Input: part model. Units: mm. Frame: model coordinates. Give positions to 0.01 mm unless a question says otherwise; leave off trailing zeros. Answer in a Markdown table with one row per item. Add a question column.
1. Ray query, line 1 (Y direction, x = -75, z = 11.5); line 2 (Z direction, x = -66, y = -19); line 3 (X direction, y = 1, z = 3.5). Return the intervals inside material, ascending. Write a range as [from, to].
2. Mould query, pull axis X, two halves, no side actions, for faces 1 (the face through (110, 5, 2)), 2 (the face through (-3, -40, 0)). Classes: released by +X, released by -X, zero draft, split by the parting line, or undercut.
3. Contact query for flat-ended pins moving along their axis: pin 1 (1.5 mm diameter, centred on x = -92, y = -22.5, fed in from +Z); pin 2 (8 mm diameter, centred on x = 65, z = -77.5, fed in from +Y); pin 3 (10 mm diameter, centred on x = -88, y = -4, fed in from +Z). Output: stop coordinate, or through.
```python
from build123d import *


with BuildPart() as part:
    # 草图2 → 放样1 section 0
    with BuildSketch(Plane(origin=(0, 0, 0), x_dir=(1, 0, 0), z_dir=(0, 1, 0))):
        with BuildLine():
            Line((-115, -115), (-115, 115))
            Line((-115, 115), (115, 115))
            Line((115, 115), (115, -115))
            Line((115, -115), (-115, -115))
        make_face()
    # 草图3 → 放样1 section 1
    with BuildSketch(Plane(origin=(0, -40, 0), x_dir=(1, 0, 0), z_dir=(0, 1, 0))):
        with BuildLine():
            Line((125, -125), (125, 125))
            Line((125, 125), (-125, 125))
            Line((-125, 125), (-125, -125))
            Line((-125, -125), (125, -125))
        make_face()
    loft()

    # 扫描1: sweep along a path in 草图2<2>
    with BuildLine(Plane(origin=(0, 0, 0), x_dir=(1, 0, 0), z_dir=(0, 1, 0))) as sweep_1_path:
        Line((-115, -115), (-115, 115))
        Line((-115, 115), (115, 115))
        Line((115, 115), (115, -115))
        Line((115, -115), (-115, -115))
    # 草图4 → 扫描1 (sweep)
    with BuildSketch(Plane(origin=(0, 0, 115), x_dir=(-1, 0, 0), z_dir=(0, 0, -1))):
        with BuildLine():
            Line((-115, 0), (-105, 0))
            ThreePointArc((-105, 0), (-110, 5), (-115, 0))
        make_face()
    sweep(path=sweep_1_path.line, transition=Transition.RIGHT)


solid = part.part
```
Answer:
| question | item | result |
|---|---|---|
| 1 | line 1 | y = [-40, 0] |
| 1 | line 2 | z = [-119.75, 119.75] |
| 1 | line 3 | x = [-114.9, -105.1], [105.1, 114.9] |
| 2 | face 1 | undercut |
| 2 | face 2 | zero draft |
| 3 | pin 1 | stops at z = 120.81 |
| 3 | pin 2 | stops at y = 0 |
| 3 | pin 3 | stops at z = 117.25 |
